Geometry check sheet. Reference: the model listing, model coordinates, mm. Face numbers are marked on the shaded views. A direction names the side the tool comes from. Give positions to 0.01 mm unless a question says otherwise; leave off trailing zeros. Write each loop counter-clockwise with the first axis right and the second up, starting at its lowest first coordinate (ties: lowest second). Pieces come first, ordered by that corner, then holes. Notation, with made-up numbers: (75, 66.25) - (79, 66.25) arc R10 ccw to (79, 73.25) - close; hole circle Ø2 at (-14.75, 14.25). An arc over 180 degrees is marked (long way). Use a Markdown table: item, result.
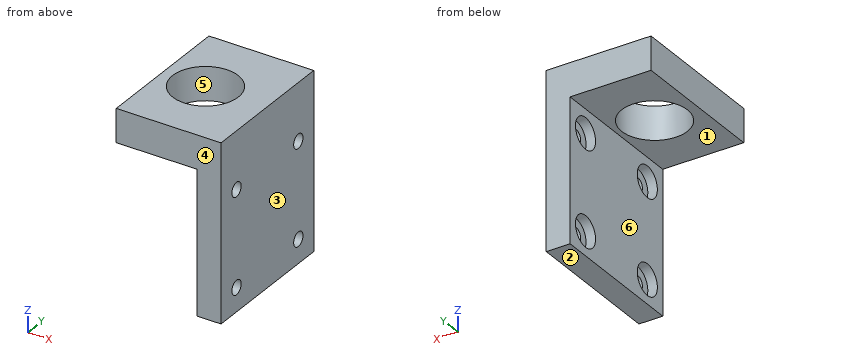
```python
from build123d import *

# Parameters (mm, degrees)
F0_W     = 22
F0_H     = 30
F1_DEPTH = 7
F2_R     = 6.9
F3_DEPTH = 25
F4_W     = 5
F4_H     = 30
F5_DEPTH = 30
F6_R     = 1.5
F7_DEPTH = 25
F8_R     = 3.25
F9_DEPTH = 2


with BuildPart() as f1:
    # F0 (on Top) → F1 (new body)
    with BuildSketch(Plane.XY):
        with Locations((11, 15)):
            Rectangle(F0_W, F0_H)
    extrude(amount=F1_DEPTH)

    # F2 (on face) → F3 (cut)
    with BuildSketch(Plane.XY.offset(7)):
        with Locations((9, 15)):
            Circle(F2_R)
    extrude(amount=-F3_DEPTH, mode=Mode.SUBTRACT)

    # F4 (on face) → F5 (join)
    with BuildSketch(Plane(origin=(0, 0, 0), x_dir=(1, 0, 0), z_dir=(0, 0, -1))):
        with Locations((19.5, -15)):
            Rectangle(F4_W, F4_H)
    extrude(amount=F5_DEPTH)

    # F6 (on face) → F7 (cut)
    with BuildSketch(Plane.YZ.offset(22)):
        with Locations((5, -25)):
            Circle(F6_R)
        with Locations((25, -25)):
            Circle(F6_R)
        with Locations((25, -5)):
            Circle(F6_R)
        with Locations((5, -5)):
            Circle(F6_R)
    extrude(amount=-F7_DEPTH, mode=Mode.SUBTRACT)

    # F8 (on face) → F9 (cut)
    with BuildSketch(Plane(origin=(17, 0, 0), x_dir=(0, -1, 0), z_dir=(-1, 0, 0))):
        with Locations((-25, -5)):
            Circle(F8_R)
        with Locations((-5, -5)):
            Circle(F8_R)
        with Locations((-5, -25)):
            Circle(F8_R)
        with Locations((-25, -25)):
            Circle(F8_R)
    extrude(amount=-F9_DEPTH, mode=Mode.SUBTRACT)


solid = f1.part
```
1) Material ranges on L1, parallel to Z at x = 17.65, y = 25; L2, parallel to Z at x = 20.45, y = 25; L3, parallel to Y at x = 9, z = 2, recorded low to high. Write a range as from..to.
Working result:
| item | result |
|---|---|
| L1 | z = -30..-28.25, -21.75..-8.25, -1.75..7 |
| L2 | z = -30..-26.5, -23.5..-6.5, -3.5..7 |
| L3 | y = 0..8.1, 21.9..30 |
2) Section check C-C on y = 25. Record the boundary of the cut face in (x, z), then the cut area to 3 significant figures.
Working result:
| item | result |
|---|---|
| outline | (0, 0) - (17, 0) - (17, -1.75) - (19, -1.75) - (19, -3.5) - (22, -3.5) - (22, 7) - (0, 7) - close; (17, -30) - (22, -30) - (22, -26.5) - (19, -26.5) - (19, -28.25) - (17, -28.25) - close; (17, -21.75) - (19, -21.75) - (19, -23.5) - (22, -23.5) - (22, -6.5) - (19, -6.5) - (19, -8.25) - (17, -8.25) - close |
| area | 260 mm² |
3) Set-up check for the marked faces 1 and 2: record each of +Z, -Z, +X, -X, +Y, -Y from which the full face is reachable in a straight line by a thin tool's end or side.
Working result:
| item | result |
|---|---|
| face 1 | -Z, -X, +Y, -Y |
| face 2 | -Z, +X, -X, +Y, -Y |
4) Section check A-A on z = -25. Record the boundary of the cut face in (x, y).
Working result:
| item | result |
|---|---|
| outline | (17, 0) - (22, 0) - (22, 3.5) - (19, 3.5) - (19, 1.75) - (17, 1.75) - close; (17, 8.25) - (19, 8.25) - (19, 6.5) - (22, 6.5) - (22, 23.5) - (19, 23.5) - (19, 21.75) - (17, 21.75) - close; (17, 28.25) - (19, 28.25) - (19, 26.5) - (22, 26.5) - (22, 30) - (17, 30) - close |
5) Section check D-D on x = 12. Record the boundary of the cut face in (y, z), then the cut area to 3 significant figures.
Working result:
| item | result |
|---|---|
| outline | (0, 0) - (8.79, 0) - (8.79, 7) - (0, 7) - close; (21.21, 0) - (30, 0) - (30, 7) - (21.21, 7) - close |
| area | 123 mm² |
6) Section check B-B on y = 15. Record the boundary of the cut face in (x, z).
Working result:
| item | result |
|---|---|
| outline | (0, 0) - (2.1, 0) - (2.1, 7) - (0, 7) - close; (15.9, 0) - (17, 0) - (17, -30) - (22, -30) - (22, 7) - (15.9, 7) - close |
7) Mould release check, pull along X, two halves, no side actions. Record for the marked faces 3, 4, 5 and 6: pulls with the +X half, pulls with the -X half, needs draft (parallel to the pull), parting line crosses it, or undercut.
Working result:
| item | result |
|---|---|
| face 3 | pulls with the +X half |
| face 4 | needs draft |
| face 5 | undercut |
| face 6 | pulls with the -X half |
8) Depth check by flat-ended pin: P1, Ø4, axis at y = 25, z = -25, coming from the +X side; P2, Ø11, axis at x = 9, y = 15, coming from the +Z side; P3, Ø7, axis at y = 6, z = -25.5, coming from the -X side; P4, Ø2, axis at y = 23.5, z = -5.5, coming from the -X side. Enter the tip coordinate at first touch or a pass-through.
Working result:
| item | result |
|---|---|
| P1 | stops at x = 22 |
| P2 | passes through |
| P3 | stops at x = 17 |
| P4 | stops at x = 19 |
